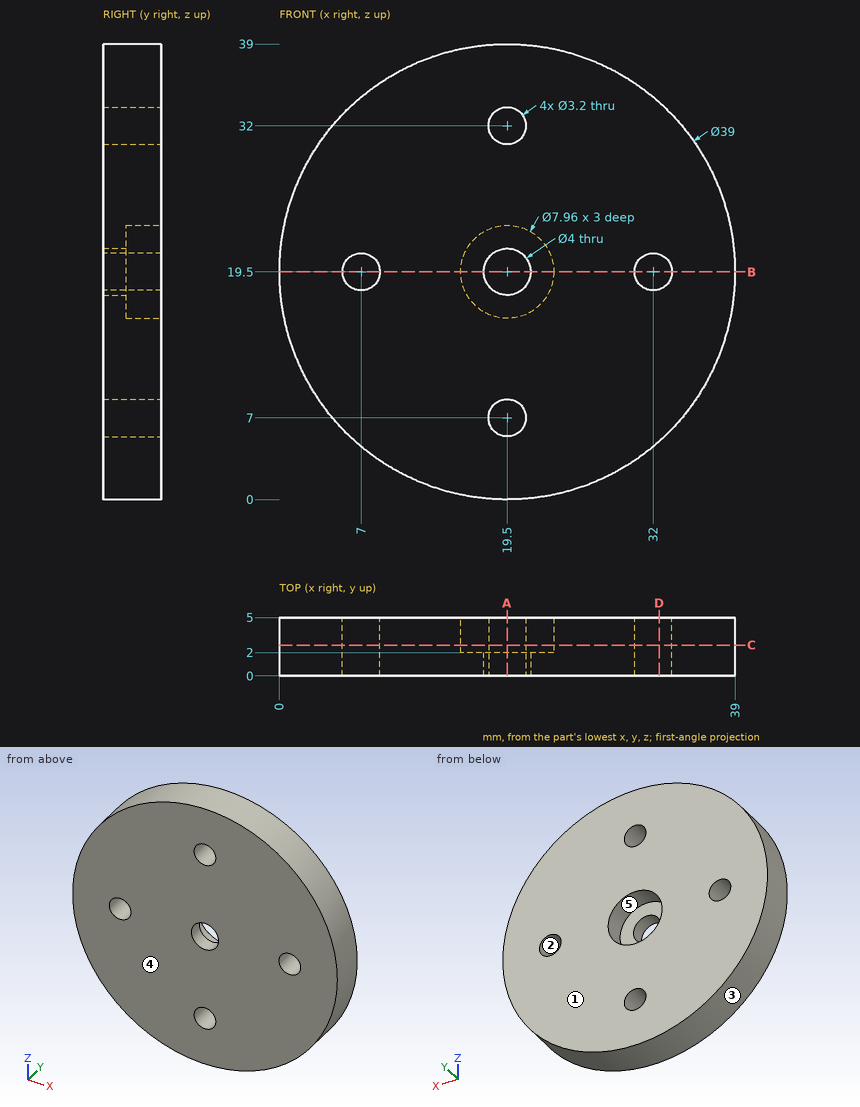
Answer from the drawing. Dimensions are ordinates in mm from the lowest x, y and z of the part. A direction names the side the tool comes from. Round coordinates to 2 decimals unless told otherwise and drop trailing zeros. Order: outer loops, then holes, each group sorted by start corner. A loop starts at its lowest first (then second) coordinate and runs counter-clockwise, first axis right, second up.
1) For the marked faces 4 and 5, determine the directions among +Z, -Z, +X, -X, +Y, -Y from which every point of the face is accessible in a straight line to the end or side of a thin tool.
2) The part is cut by section B-B on z = 19.5. Write down the section's boundary in (x, y).
3) Straight lines are drawn through the part: L1, parallel to Z at x = 19.5, y = 2.95; L2, parallel to Z at x = 19.5, y = 1.15. For each, find the intervals that lie inside material, in ascending order.
4) The mould has two halves that part along X. Classify the marked faces 1, 2 and 3: released by +X, released by -X, zero draft, split by the parting line, or undercut.
5) The part is cut by section A-A on x = 19.5. Write down the section's boundary in (y, z).
6) Flat-ended cylindrical pins translate along their axes: pin 1 (4 mm diameter, centred on x = 19.5, z = 18.5, fed in from +Y); pin 2 (3 mm diameter, centred on x = 21.5, y = 0.5, fed in from +Z); pin 3 (1 mm diameter, centred on y = 4, z = 24.5, fed in from +X). Find the tip coordinate at first contact, or state that the pin passes through.
7) The part is cut by section C-C on y = 2.65. Write down the section's boundary in (x, z).
8) The part is cut by section D-D on x = 32.5. Write down the section's boundary in (y, z).
Resolved:
1. face 4: +Z, -Z, +X, -X, -Y
1. face 5: +Y
2. outline: (0, 0) - (5.4, 0) - (5.4, 5) - (0, 5) - close; (8.6, 0) - (17.5, 0) - (17.5, 2) - (15.52, 2) - (15.52, 5) - (8.6, 5) - close; (21.5, 0) - (30.4, 0) - (30.4, 5) - (23.48, 5) - (23.48, 2) - (21.5, 2) - close; (33.6, 0) - (39, 0) - (39, 5) - (33.6, 5) - close
3. L1: z = 0 to 5.4, 8.6 to 15.52, 23.48 to 30.4, 33.6 to 39
3. L2: z = 0 to 5.4, 8.6 to 17.5, 21.5 to 30.4, 33.6 to 39
4. face 1: zero draft
4. face 2: undercut
4. face 3: split by the parting line
5. outline: (0, 0) - (5, 0) - (5, 5.4) - (0, 5.4) - close; (0, 8.6) - (5, 8.6) - (5, 15.52) - (2, 15.52) - (2, 17.5) - (0, 17.5) - close; (0, 21.5) - (2, 21.5) - (2, 23.48) - (5, 23.48) - (5, 30.4) - (0, 30.4) - close; (0, 33.6) - (5, 33.6) - (5, 39) - (0, 39) - close
6. pin 1: stops at y = 2
6. pin 2: stops at z = 38.99
6. pin 3: stops at x = 38.47
7. outline: circle Ø39 at (19.5, 19.5); hole circle Ø3.2 at (7, 19.5); hole circle Ø7.96 at (19.5, 19.5); hole circle Ø3.2 at (19.5, 7); hole circle Ø3.2 at (19.5, 32); hole circle Ø3.2 at (32, 19.5)
8. outline: (0, 4.97) - (5, 4.97) - (5, 17.98) - (0, 17.98) - close; (0, 21.02) - (5, 21.02) - (5, 34.03) - (0, 34.03) - close
